from build123d import *

# Parameters (mm, degrees)
SKETCH1_W           = 120
SKETCH1_H           = 30
BOSS_EXTRUDE1_DEPTH = 165
SKETCH2_R           = 4
CUT_EXTRUDE1_DEPTH  = 331


with BuildPart() as part:
    # Sketch1 → Boss-Extrude1 (new body, symmetric)
    with BuildSketch(Plane.XY):
        Rectangle(SKETCH1_W, SKETCH1_H)
    extrude(amount=BOSS_EXTRUDE1_DEPTH, both=True)

    # Sketch2 → Cut-Extrude1 (cut, through all)
    with BuildSketch(Plane(origin=(0, 0, -165), x_dir=(-1, 0, 0), z_dir=(0, 0, -1))):
        with Locations((-45, 0)):
            Circle(SKETCH2_R)
        with Locations((-15, 0)):
            Circle(SKETCH2_R)
        with Locations((15, 0)):
            Circle(SKETCH2_R)
        with Locations((45, 0)):
            Circle(SKETCH2_R)
    extrude(amount=-CUT_EXTRUDE1_DEPTH, mode=Mode.SUBTRACT)


solid = part.part
Can you work these out from the model? Positions are in its coordinate system, mm. Coordinates: 2 decimals unless noted, no trailing zeros. Loops run counter-clockwise (first coordinate to the right, second up) from the corner with the lowest first, then second, coordinate; pieces in that order, holes last. Notation, with made-up numbers: M 66,-0.75 L 70,-0.75 A11 cw 70,18.25 Z; hole C 14.5,85.5 d11. An arc over 180 degrees is marked long. Answer as CSV lines item,"result". Start each with the question number.
1. For pin 1 Ø10.5 at (x, y) = (-15, 0) entering from +Z, with a flat end and sliding along its axis, tell me the tip position at first contact or that it passes through.
2. Thinking about a two-plate mould opening in X: for faces 1 (the face through (-1, 0, 165)), 2 (the face through (-41.8, -2.4, -2.3)), 3 (the face through (60, 0, 2)), which applies, +X half, -X half, draft (parallel to the pull), parting line (faces both ways), or undercut?
3. Suppose I cut it at A-A, the plane x = 45. List the corners of the cut face in (y, z) for me, plus the area to 3 significant figures.
4. If I drill on probe 1 along Y at (x, z) = (15, 73); probe 2 along X at (y, z) = (1.5, 67); probe 3 along X at (y, z) = (-1.75, -1), over which ranges is the centre line in solid material (lowest first)? Write a range as [from, to].
5. Suppose I cut it at B-B, the plane y = 0. List the corners of the cut face in (x, z) for me, plus the area to 3 significant figures.
6. Suppose I cut it at C-C, the plane z = -41. List the corners of the cut face in (x, y) for me, plus the area to 3 significant figures.
Output:
1,pin 1,"stops at z = 165"
2,face 1,"draft"
2,face 2,"undercut"
2,face 3,"+X half"
3,outline,"M -15,-165 L -4,-165 L -4,165 L -15,165 Z; M 4,-165 L 15,-165 L 15,165 L 4,165 Z"
3,area,"7,260 mm^2"
4,probe 1,"y = [-15, -4], [4, 15]"
4,probe 2,"x = [-60, -48.71], [-41.29, -18.71], [-11.29, 11.29], [18.71, 41.29], [48.71, 60]"
4,probe 3,"x = [-60, -48.6], [-41.4, -18.6], [-11.4, 11.4], [18.6, 41.4], [48.6, 60]"
5,outline,"M -60,-165 L -49,-165 L -49,165 L -60,165 Z; M -41,-165 L -19,-165 L -19,165 L -41,165 Z; M -11,-165 L 11,-165 L 11,165 L -11,165 Z; M 19,-165 L 41,-165 L 41,165 L 19,165 Z; M 49,-165 L 60,-165 L 60,165 L 49,165 Z"
5,area,"29,000 mm^2"
6,outline,"M -60,-15 L 60,-15 L 60,15 L -60,15 Z; hole C -45,0 d8; hole C -15,0 d8; hole C 15,0 d8; hole C 45,0 d8"
6,area,"3,400 mm^2"
